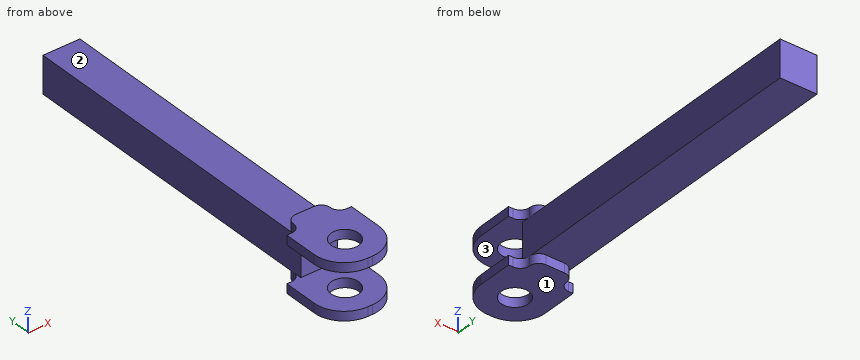
```python
from build123d import *

# Parameters (mm, degrees)
SKETCH1_W           = 50.8
SKETCH1_H           = 50.8
BOSS_EXTRUDE1_DEPTH = 450
SKETCH3_R           = 19.05
BOSS_EXTRUDE2_DEPTH = 12.7
FILLET1_R           = 12.7
FILLET3_R           = 41.275


with BuildPart() as part:
    # Sketch1 → Boss-Extrude1 (new body)
    with BuildSketch(Plane(origin=(0, 0, 0), x_dir=(1, 0, 0), z_dir=(0, 1, 0))):
        Rectangle(SKETCH1_W, SKETCH1_H)
    extrude(amount=BOSS_EXTRUDE1_DEPTH)

    # Sketch3 → Boss-Extrude2 (add)
    with BuildSketch(Plane.XY.offset(25.4)):
        Polygon((-25.4, 0), (-25.4, 25.4), (25.4, 25.4), (25.4, 0), (44.45, 0), (44.45, -88.9), (-44.45, -88.9), (-44.45, 0), align=None)
        with Locations((0, -45)):
            Circle(SKETCH3_R, mode=Mode.SUBTRACT)
    boss_extrude2 = extrude(amount=BOSS_EXTRUDE2_DEPTH)

    # Mirror1: Boss-Extrude2 across plane
    add(boss_extrude2.mirror(Plane.XY))

    # Fillet1
    fillet1_edges = [part.edges().sort_by_distance(p)[0] for p in [
        (25.4, 0, 31.75),
        (25.4, 0, -31.75),
        (-25.4, 0, -31.75),
        (-25.4, 0, 31.75),
    ]]
    fillet(fillet1_edges, radius=FILLET1_R)
    fillet1_2_edges = [part.edges().sort_by_distance(p)[0] for p in [
        (25.4, 25.4, -31.75),
        (-25.4, 25.4, -31.75),
        (25.4, 25.4, 31.75),
        (-25.4, 25.4, 31.75),
    ]]
    fillet(fillet1_2_edges, radius=FILLET1_R - 0.0001)  # a hair under: the kernel refuses the full size

    # Fillet3
    fillet3_edges = [part.edges().sort_by_distance(p)[0] for p in [
        (-44.45, -88.9, 31.75),
        (44.45, -88.9, 31.75),
        (-44.45, -88.9, -31.75),
        (44.45, -88.9, -31.75),
    ]]
    fillet(fillet3_edges, radius=FILLET3_R)


solid = part.part
```
Source: CAD feature listing. Evaluate the final solid. Frame: model axes, mm. Face numbers are marked on the shaded views. Round coordinates to 2 decimals unless told otherwise and drop trailing zeros. Loops run counter-clockwise (first coordinate to the right, second up) from the corner with the lowest first, then second, coordinate; pieces in that order, holes last. Notation, with made-up numbers: M 2.25,-31 L 47.25,-31 A27 ccw 47.25,0 Z; hole C 26,42 d11. An arc over 180 degrees is marked long. Use a Markdown table: item, result. Add a question column.
1. Contact query for flat-ended pins moving along their axis: P1, Ø2, axis at y = 66.5, z = -21.5, coming from the -X side; P2, Ø7, axis at x = 42, z = -31, coming from the +Y side; P3, Ø8, axis at y = 276, z = 23, coming from the +X side. Output: stop coordinate, or through.
2. Section query B-B on z = 2.5. Return the cut outline in (x, y), then the cut area to 3 significant figures.
3. Mould query, pull axis Z, two halves, no side actions, for the marked faces 1, 2 and 3. Classes: pulls with the +Z half, pulls with the -Z half, needs draft (parallel to the pull), parting line crosses it, or undercut.
4. Line query: line 1 (Y direction, x = 0, z = 29.5); line 2 (Z direction, x = -9.5, y = 164); line 3 (Y direction, x = -10, z = -2). Output: solid intervals per line, ascending.
5. Section query A-A on y = 128. Return the cut outline in (x, z), then the cut area to 3 significant figures.
Reported:
| question | item | result |
|---|---|---|
| 1 | P1 | stops at x = -25.4 |
| 1 | P2 | stops at y = 0 |
| 1 | P3 | stops at x = 25.4 |
| 2 | outline | M -25.4,0 L 25.4,0 L 25.4,450 L -25.4,450 Z |
| 2 | area | 22,900 mm² |
| 3 | face 1 | pulls with the -Z half |
| 3 | face 2 | pulls with the +Z half |
| 3 | face 3 | undercut |
| 4 | line 1 | y = -88.9 to -64.05, -25.95 to 25.4 |
| 4 | line 2 | z = -25.4 to 25.4 |
| 4 | line 3 | y = 0 to 450 |
| 5 | outline | M -25.4,-25.4 L 25.4,-25.4 L 25.4,25.4 L -25.4,25.4 Z |
| 5 | area | 2,580 mm² |
